Check sheet for the drawn part. Datum: minimum x, y, z corner. Units: mm. A direction names the side the tool comes from. Give positions to 0.01 mm unless a question says otherwise; leave off trailing zeros. Order: outer loops, then holes, each group sorted by start corner. A loop starts at its lowest first (then second) coordinate and runs counter-clockwise, first axis right, second up. Notation, with made-up numbers: (64, 49.25) - (85, 49.25) arc R32 cw to (85, 78.25) - close; hole circle Ø9 at (74, 81.5). An arc over 180 degrees is marked (long way). Answer as a JSON object with one key per item and string values. Group by question number.
(1) Thickness scan on line 1 (Y direction, x = 23, z = 14); line 2 (X direction, y = 28, z = 19.5); line 3 (Y direction, x = 36, z = 40) (3 decimals). Record the ranges inside material, lowest first.
(2) Section check B-B (y = 58). Record the boundary of the cut face in (x, z).
(3) Depth check by flat-ended pin: pin 1 Ø10 at (x, z) = (47.5, 19) entering from -Y; pin 2 Ø4 at (x, y) = (38.5, 38.5) entering from +Z; pin 3 Ø1 at (x, z) = (39, 32) entering from -Y (3 decimals). Enter the tip coordinate at first touch or a pass-through.
(4) Section check C-C (x = 10.5). Record the boundary of the cut face in (y, z).
(5) Section check D-D (z = 24.5). Record the boundary of the cut face in (x, y) (3 decimals), then the cut area to 3 significant figures.
(6) Access from +Z, -Z, +X, -X, +Y, -Y to the whole of each face (thin tool, end or side, straight path). Record for the marked faces 1, 2, 3, 4 and 5.
(7) Section check A-A (z = 58). Record the boundary of the cut face in (x, y) (3 decimals).
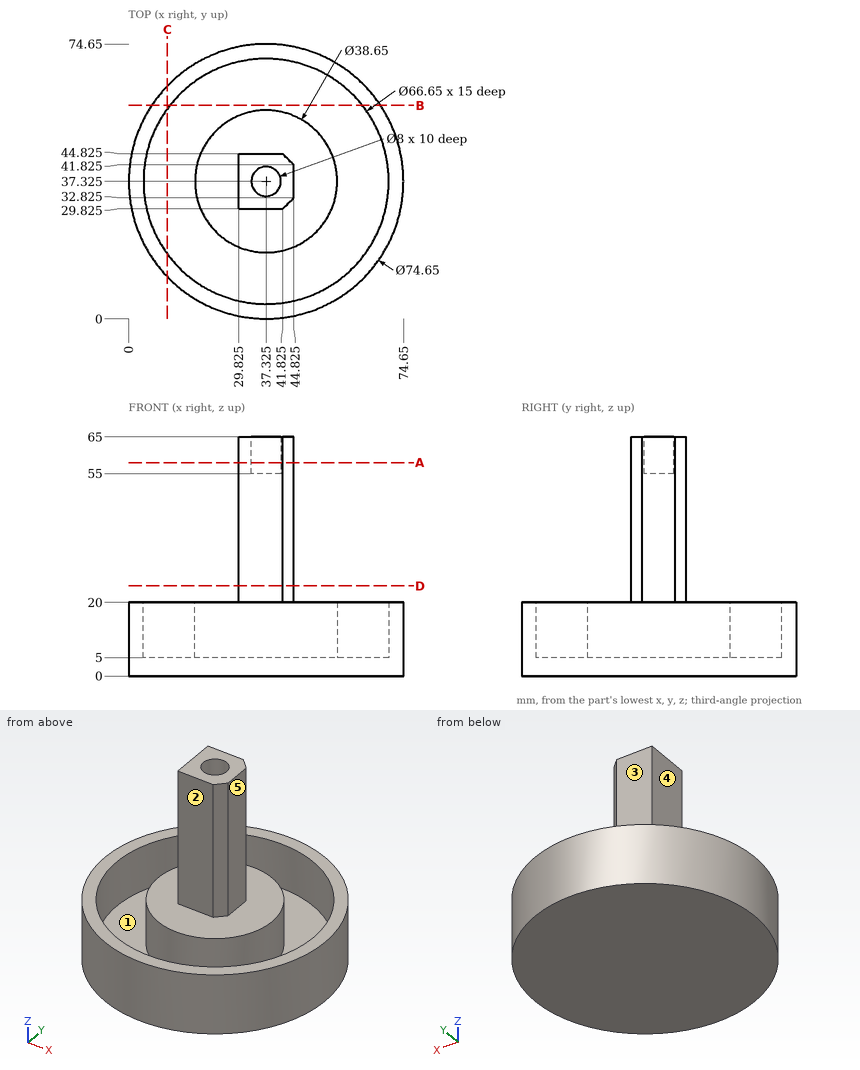
Solutions:
{
 "1": {"line 1": "y = 2.86 to 7.24, 24.35 to 50.3, 67.41 to 71.79", "line 2": "x = 1.18 to 5.33, 20.4 to 54.25, 69.32 to 73.47", "line 3": "y = 29.825 to 44.825"},
 "2": {"outline": "(6.25, 0) - (68.4, 0) - (68.4, 20) - (63.46, 20) - (63.46, 5) - (11.19, 5) - (11.19, 20) - (6.25, 20) - close"},
 "3": {"pin 1": "stops at y = 0.36", "pin 2": "stops at z = 55", "pin 3": "stops at y = 29.825"},
 "4": {"outline": "(11.37, 0) - (63.28, 0) - (63.28, 20) - (57.1, 20) - (57.1, 5) - (17.55, 5) - (17.55, 20) - (11.37, 20) - close"},
 "5": {"outline": "(29.825, 29.825) - (41.825, 29.825) - (44.825, 32.825) - (44.825, 41.825) - (41.825, 44.825) - (29.825, 44.825) - close", "area": "216 mm2"},
 "6": {"face 1": "+Z", "face 2": "+Z, +X, -X, -Y", "face 3": "+Z, +X, -X, +Y", "face 4": "+Z, -X, +Y, -Y", "face 5": "+Z, +X, +Y, -Y"},
 "7": {"outline": "(29.825, 29.825) - (41.825, 29.825) - (44.825, 32.825) - (44.825, 41.825) - (41.825, 44.825) - (29.825, 44.825) - close; hole circle Ø8 at (37.325, 37.325)"}
}
